Input: part model. Units: mm. Frame: model coordinates. Face numbers are marked on the shaded views. A direction names the side the tool comes from. Coordinates: 2 decimals unless noted, no trailing zeros. Order: outer loops, then holes, each group sorted by start corner. A loop starts at its lowest first (then second) coordinate and runs counter-clockwise, first axis right, second up. Notation, with made-up numbers: (10, 59.25) -> (35, 59.25) arc R14 cw to (35, 69.25) -> close; hole circle Ø3 at (31, 26). An arc over 180 degrees is marked (long way). One line per item, written item: value. Start each with the question number.
from build123d import *

# Parameters (mm, degrees)
F0_R      = 28.5877
F1_DEPTH  = 21.9329
F3_DEPTH  = 1.5367
F4_R      = 5.55625
F5_DEPTH  = 2.6924
F6_R      = 3.175
F7_DEPTH  = 15.8877
F8_R      = 3.53695
F9_DEPTH  = 1.9812
F10_R     = 1.3843
F11_DEPTH = 23.4706


with BuildPart() as f1:
    # F0 (on Front) → F1 (new body)
    with BuildSketch(Plane.XZ):
        Circle(F0_R)
    extrude(amount=-F1_DEPTH)

    # F2 (on face) → F3 (join)
    with BuildSketch(Plane.XZ):
        with BuildLine():
            Line((-10.604302, 19.560907), (-36.389242, 5.582451))
            ThreePointArc((-36.389242, 5.582451), (-39.7129, 0), (-36.389242, -5.582451))
            Line((-36.389242, -5.582451), (-10.604302, -19.560907))
            ThreePointArc((-10.604302, -19.560907), (0, -22.2504), (10.604302, -19.560907))
            Line((10.604302, -19.560907), (36.389242, -5.582451))
            ThreePointArc((36.389242, -5.582451), (39.7129, 0), (36.389242, 5.582451))
            Line((36.389242, 5.582451), (10.604302, 19.560907))
            ThreePointArc((10.604302, 19.560907), (0, 22.2504), (-10.604302, 19.560907))
        make_face()
    extrude(amount=F3_DEPTH)

    # F4 (on face) → F5 (join)
    with BuildSketch(Plane.XZ.offset(1.5367)):
        Circle(F4_R)
    extrude(amount=F5_DEPTH)

    # F6 (on face) → F7 (join)
    with BuildSketch(Plane.XZ.offset(4.2291)):
        Circle(F6_R)
    extrude(amount=F7_DEPTH)

    # F8 (on face) → F9 (join)
    with BuildSketch(Plane(origin=(0, 0, 0), x_dir=(-1, 0, 0), z_dir=(0, 1, 0))):
        with Locations((-33.3629, 0)):
            Circle(F8_R)
        with Locations((33.3629, 0)):
            Circle(F8_R)
    extrude(amount=F9_DEPTH)

    # F10 (on face) → F11 (cut, through all)
    with BuildSketch(Plane.XZ.offset(1.5367)):
        with Locations((33.3629, 0)):
            Circle(F10_R)
        with Locations((-33.3629, 0)):
            Circle(F10_R)
    extrude(amount=-F11_DEPTH, mode=Mode.SUBTRACT)


solid = f1.part
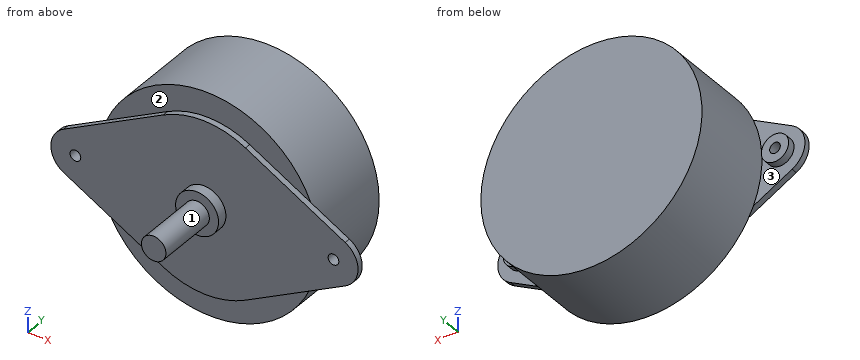
1) Section query A-A, the plane z = 0. State how many separate pieces and enclosed holes the cut face has, plus the area to 3 significant figures.
2) Access query for the marked faces 1, 2 and 3. Directions: +Z, -Z, +X, -X, +Y, -Y. A direction counts if a zero-diameter tool reaches every point of the face in a straight line with its end or side. Return the directions, or none.
3) Section query C-C, the plane y = 5. Return the cut outline in (x, z), plus the area to 3 significant figures.
4) Section query B-B, the plane x = 0. Return the cut outline in (y, z) (3 decimals).
5) Ray query, line 1 along Y through (x, z) = (-16.5, 5); line 2 along Y through (x, z) = (5.5, -23); line 3 along Z through (x, y) = (-11, 0.5). Return the intervals inside material, ascending. Write a range as from..to.
6) Section query D-D, the plane x = 9. Return the cut outline in (y, z).
7) Pin query (flat end, axial travel): pin 1 Ø14.5 at (x, z) = (-32, -1.5) entering from +Y; pin 2 Ø5.5 at (x, z) = (-35, -1.5) entering from +Y; pin 3 Ø4.5 at (x, z) = (-33.36, 0) entering from -Y; pin 4 Ø4 at (x, y) = (23, -3) entering from +Z. Return the tip coordinate at first contact, or that it passes through.
Entries:
1. separate pieces: 3
1. enclosed holes: 0
1. area: 1,520 mm2
2. face 1: -Y
2. face 2: +Z, -Y
2. face 3: +Y
3. outline: circle Ø57.18 at (0, 0)
3. area: 2,570 mm2
4. outline: (-20.117, -3.175) -> (-4.229, -3.175) -> (-4.229, -5.556) -> (-1.537, -5.556) -> (-1.537, -22.25) -> (0, -22.25) -> (0, -28.588) -> (21.933, -28.588) -> (21.933, 28.588) -> (0, 28.588) -> (0, 22.25) -> (-1.537, 22.25) -> (-1.537, 5.556) -> (-4.229, 5.556) -> (-4.229, 3.175) -> (-20.117, 3.175) -> close
5. line 1: y = -1.54..21.93
5. line 2: y = 0..21.93
5. line 3: z = -26.39..26.39
6. outline: (-1.54, -20.35) -> (0, -20.35) -> (0, -27.13) -> (21.93, -27.13) -> (21.93, 27.13) -> (0, 27.13) -> (0, 20.35) -> (-1.54, 20.35) -> close
7. pin 1: stops at y = 21.93
7. pin 2: stops at y = 1.98
7. pin 3: stops at y = -1.54
7. pin 4: stops at z = 13.58
